Build history of the part. All positions in model axes, mm. Face numbers are marked on the shaded views. A direction names the side the tool comes from. Give positions to 0.01 mm unless a question says otherwise; leave off trailing zeros. Loops run counter-clockwise (first coordinate to the right, second up) from the corner with the lowest first, then second, coordinate; pieces in that order, holes last.
1) 3-axis set-ups, long thin cutter, end or side, ignore diameter. For the marked faces 1 and 2: which of +Z, -Z, +X, -X, +Y, -Y reach the whole face in a straight line?
2) Band-saw the part on C-C on x = -74.5. List the corners of the cut face in (y, z), then the cut area to 3 significant figures.
3) Band-saw the part on A-A on z = 10. List the corners of the cut face in (x, y), then the cut area to 3 significant figures.
4) Flat gauge pins, fed straight in: P1, Ø8, axis at y = -119, z = 11.5, coming from the +X side; P2, Ø4.5, axis at x = -130, y = -121, coming from the -Z side; P3, Ø5, axis at x = -107, z = 11, coming from the +Y side. Where does each tip first touch, or does it go through?
5) Band-saw the part on B-B on y = -123. List the corners of the cut face in (x, z), then the cut area to 3 significant figures.
6) Wall check: line 1 (X direction, y = -110, z = 5.5); line 2 (Y direction, x = -138, z = 10.25); line 3 (Y direction, x = -25.5, z = 11.25). Give the ranges that are in metal, low to high.
7) Band-saw the part on D-D on y = -96.5. List the corners of the cut face in (x, z), then the cut area to 3 significant figures.
```python
from build123d import *

# Parameters (mm, degrees)
BOSS_EXTRUDE1_DEPTH = 20
SKETCH6_W           = 5
SKETCH6_H           = 20
CUT_EXTRUDE1_DEPTH  = 293.280687012
SKETCH7_R           = 1.5
BOSS_EXTRUDE2_DEPTH = 15
BOSS_EXTRUDE3_START = 15
SKETCH8_R           = 1.5
BOSS_EXTRUDE3_DEPTH = 15
SKETCH9_W           = 68.096715613
SKETCH9_H           = 158.263972947
CUT_EXTRUDE2_DEPTH  = 153
SKETCH10_W          = 29.496800943
SKETCH10_H          = 9.142322102
CUT_EXTRUDE3_DEPTH  = 20


with BuildPart() as part:
    # Sketch5 → Boss-Extrude1 (new body)
    with BuildSketch(Plane.XY):
        Polygon((0, 0), (-42.5, 0), (-131, -108), (-131, -128), (-128, -128), (-128, -109.072168564), (-41.07975076, -3), (0, -3), align=None)
        Polygon((42.5, 0), (0, 0), (0, -3), (41.07975076, -3), (128, -109.072168564), (128, -128), (131, -128), (131, -108), align=None)
    extrude(amount=BOSS_EXTRUDE1_DEPTH)

    # Sketch6 → Cut-Extrude1 (cut, through all)
    with BuildSketch(Plane(origin=(131, 0, 0), x_dir=(0, 0, -1), z_dir=(1, 0, 0))):
        with Locations((-17.5, -118)):
            Rectangle(SKETCH6_W, SKETCH6_H)
        Polygon((-20, -108), (-15, -108), (-20, 0), align=None)
        Polygon((0, 0), (-5, -108), (0, -108), align=None)
        with Locations((-2.5, -118)):
            Rectangle(SKETCH6_W, SKETCH6_H)
    extrude(amount=-CUT_EXTRUDE1_DEPTH, mode=Mode.SUBTRACT)

    # Sketch7 → Boss-Extrude2 (add)
    with BuildSketch(Plane(origin=(131, 0, 0), x_dir=(0, 0, -1), z_dir=(1, 0, 0))):
        with Locations((-10, -123)):
            Circle(SKETCH7_R)
    extrude(amount=BOSS_EXTRUDE2_DEPTH)

    # Sketch8 → Boss-Extrude3 (add)
    with BuildSketch(Plane.ZY.offset(131).offset(BOSS_EXTRUDE3_START)):
        with Locations(Location((10, -123, 0), (0, 0, 180))):
            Circle(SKETCH8_R)
    extrude(amount=-BOSS_EXTRUDE3_DEPTH)

    # Sketch9 → Cut-Extrude2 (cut)
    with BuildSketch(Plane(origin=(0, 0, 0), x_dir=(0, 0, -1), z_dir=(1, 0, 0))):
        with Locations((10.702862104, -71.494594105)):
            Rectangle(SKETCH9_W, SKETCH9_H)
    extrude(amount=CUT_EXTRUDE2_DEPTH, mode=Mode.SUBTRACT)

    # Sketch10 → Cut-Extrude3 (cut)
    with BuildSketch(Plane(origin=(0, 0, 0), x_dir=(0, 0, -1), z_dir=(1, 0, 0))):
        with Locations((-8.497508997, -2.151596762)):
            Rectangle(SKETCH10_W, SKETCH10_H)
    extrude(amount=-CUT_EXTRUDE3_DEPTH, mode=Mode.SUBTRACT)


solid = part.part
```
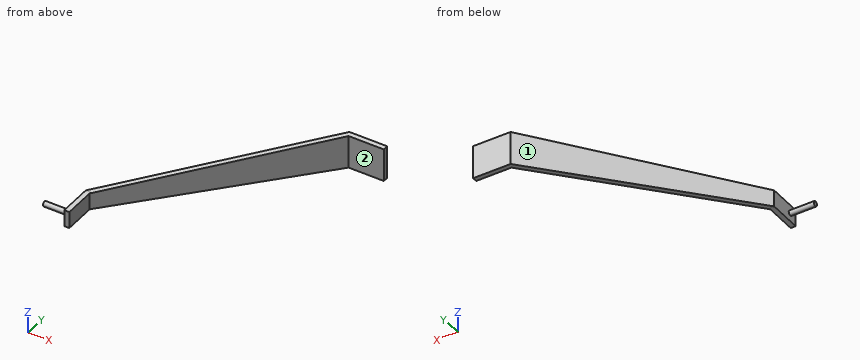
Findings below:
1. face 1: +Z, -Z, -X, +Y
1. face 2: +Z, -Z, +X, -Y
2. outline: (-43.78, 2.03) - (-39.05, 1.81) - (-39.05, 18.19) - (-43.78, 17.97) - close
2. area: 76.5 mm2
3. outline: (-146, -124.5) - (-131, -124.5) - (-131, -128) - (-128, -128) - (-128, -109.07) - (-41.08, -3) - (-20, -3) - (-20, 0) - (-42.5, 0) - (-131, -108) - (-131, -121.5) - (-146, -121.5) - close
3. area: 584 mm2
4. P1: stops at x = -128
4. P2: stops at z = 5
4. P3: stops at y = -75.66
5. outline: (-146, 8.5) - (-131, 8.5) - (-131, 5) - (-128, 5) - (-128, 15) - (-131, 15) - (-131, 11.5) - (-146, 11.5) - close
5. area: 75.0 mm2
6. line 1: x = -131 to -128
6. line 2: y = -124.48 to -121.52
6. line 3: y = -3 to 0
7. outline: (-121.58, 4.47) - (-117.7, 4.47) - (-117.7, 15.53) - (-121.58, 15.53) - close
7. area: 42.9 mm2
